Autodesk Inventor part; units mm, degrees
ref_plane "YZ Plane" through (0, 0, 0) normal (1, 0, 0) x (0, 1, 0)
ref_plane "XZ Plane" through (0, 0, 0) normal (0, 1, 0) x (-1, 0, 0)
ref_plane "XY Plane" through (0, 0, 0) normal (0, 0, 1) x (1, 0, 0)
sketch "Sketch1" plane through (0, 0, 0) normal (0, 0, 1) x (1, 0, 0)
  line L0 (0, 0) -> (95.25, 0)
  line L1 (95.25, 0) -> (95.25, -146.05)
  line L2 (95.25, -146.05) -> (0, -146.05)
  line L3 (0, -146.05) -> (0, 0)
  dimension "d0" = 95.25
  dimension "d1" = 146.05
extrude "Extrusion1" add sketch "Sketch1" along normal blind 6.35
sketch "Sketch2" plane through (0, 0, 6.35) normal (0, 0, 1) x (1, 0, 0)
  line L0 (95.25, 0) -> (0, 0)
  line L1 (95.25, 0) -> (-31.75, 0)
  line L2 (-31.75, 0) -> (-31.75, -6.35)
  line L3 (-31.75, -6.35) -> (95.25, -6.35)
  line L4 (95.25, -146.05) -> (95.25, 0)
  line L5 (95.25, -6.35) -> (95.25, 0)
  dimension "d4" = 127
  dimension "d5" = 6.35
extrude "Extrusion2" add sketch "Sketch2" along normal blind 203.2
sketch "Sketch3" plane through (0, 0, 209.55) normal (0, 0, 1) x (1, 0, 0)
  line L0 (0, 0) -> (95.25, 0)
  line L1 (95.25, -146.05) -> (95.25, -6.35)
  line L2 (0, 0) -> (95.25, 0)
  line L3 (95.25, 0) -> (95.25, -6.35)
  line L4 (95.25, -6.35) -> (0, -6.35)
  line L5 (0, -6.35) -> (0, 0)
extrude "Extrusion3" add sketch "Sketch3" along normal blind 6.35
sketch "Sketch4" plane through (-31.75, -6.35, 6.35) normal (0, -1, 0) x (1, 0, 0)
  line L0 (0, 203.2) -> (31.75, 203.2)
  line L1 (31.75, 209.55) -> (127, 209.55)
  line L2 (31.75, 203.2) -> (127, 203.2)
  line L3 (127, 203.2) -> (127, 209.55)
  line L4 (127, 209.55) -> (31.75, 209.55)
  line L5 (31.75, 209.55) -> (31.75, 203.2)
  point P0 (31.75, -6.35)
extrude "Extrusion4" add sketch "Sketch4" along normal blind 139.7
sketch "Sketch5" plane through (0, -146.05, 0) normal (-1, 0, 0) x (0, 0, 1)
  line L0 (0, 146.05) -> (215.9, 146.05)
  line L1 (0, 0) -> (6.35, 0)
  line L2 (0, 146.05) -> (6.35, 146.05)
  line L3 (6.35, 146.05) -> (6.35, 0)
  line L4 (6.35, 0) -> (0, 0)
  line L5 (0, 0) -> (0, 146.05)
extrude "Extrusion5" add sketch "Sketch5" along normal blind 342.9
sketch "Sketch6" plane through (0, 0, 209.55) normal (-1, 0, 0) x (0, 0, 1)
  line L0 (-209.55, 0) -> (6.35, 0)
  line L1 (0, -6.35) -> (0, -146.05)
  line L2 (6.35, 0) -> (0, 0)
  line L3 (0, 0) -> (0, -146.05)
  line L4 (0, -146.05) -> (6.35, -146.05)
  line L5 (6.35, -146.05) -> (6.35, 0)
extrude "Extrusion6" add sketch "Sketch6" along normal blind 342.9
properties part number "Gen2Plate"
Geometry check sheet. Reference: the model listing, model coordinates, mm. A direction names the side the tool comes from. Give positions to 0.01 mm unless a question says otherwise; leave off trailing zeros. Write each loop counter-clockwise with the first axis right and the second up, starting at its lowest first coordinate (ties: lowest second). Pieces come first, ordered by that corner, then holes. Notation, with made-up numbers: (24.25, 77.5) - (77.25, 77.5) arc R10 ccw to (77.25, 86.5) - close; hole circle Ø2 at (-3.5, -37.5). An arc over 180 degrees is marked (long way). Use a Markdown table: item, result.
Q1. Section check D-D, the plane z = 92.5. Enter the section's corners in (x, y), then the cut area to 3 significant figures.
Computed:
| item | result |
|---|---|
| outline | (-31.75, -6.35) - (95.25, -6.35) - (95.25, 0) - (-31.75, 0) - close |
| area | 806 mm² |
Q2. Section check C-C, the plane x = 54. Enter the section's corners in (y, z).
Computed:
| item | result |
|---|---|
| outline | (-146.05, 0) - (0, 0) - (0, 215.9) - (-146.05, 215.9) - (-146.05, 209.55) - (-6.35, 209.55) - (-6.35, 6.35) - (-146.05, 6.35) - close |
Q3. Draft check along Z on faces 1 (the face through (95.25, -2, 107)), 2 (the face through (-121, -74, 215.9)), 3 (the face through (-121, -72, 6.35)). Enter one of: pulls with the +Z half, pulls with the -Z half, needs draft (parallel to the pull), parting line crosses it, or undercut.
Computed:
| item | result |
|---|---|
| face 1 | needs draft |
| face 2 | pulls with the +Z half |
| face 3 | undercut |
Q4. Set-up check for faces 4 (the face through (33, -6.35, 107)), 5 (the face through (-121, -74, 0)): record each of +Z, -Z, +X, -X, +Y, -Y from which the full face is reachable in a straight line by a thin tool's end or side.
Computed:
| item | result |
|---|---|
| face 4 | +X, -X, -Y |
| face 5 | -Z, +X, -X, +Y, -Y |
Q5. Go/stop test with a flat-tipped pin: P1, Ø1.9, axis at y = -2, z = 149.5, coming from the -X side. Record where the tip stops, or that it passes through.
Computed:
| item | result |
|---|---|
| P1 | stops at x = -31.75 |
Q6. Section check A-A, the plane x = -44. Enter the section's corners in (y, z).
Computed:
| item | result |
|---|---|
| outline | (-146.05, 0) - (0, 0) - (0, 6.35) - (-146.05, 6.35) - close; (-146.05, 209.55) - (0, 209.55) - (0, 215.9) - (-146.05, 215.9) - close |
Q7. Section check B-B, the plane y = -75. Enter the section's corners in (x, z).
Computed:
| item | result |
|---|---|
| outline | (-342.9, 0) - (95.25, 0) - (95.25, 6.35) - (-342.9, 6.35) - close; (-342.9, 209.55) - (95.25, 209.55) - (95.25, 215.9) - (-342.9, 215.9) - close |
Q8. Thickness scan on L1, parallel to Z at x = -207.5, y = -135.5; L2, parallel to Y at x = 61, z = 163. Record the ranges inside material, lowest first. Write a range as [from, to].
Computed:
| item | result |
|---|---|
| L1 | z = [0, 6.35], [209.55, 215.9] |
| L2 | y = [-6.35, 0] |
